Could you check a few things on this model? Use its own coordinates, in mm. A direction names the side the tool comes from. Coordinates: 2 decimals unless noted, no trailing zeros. Loops run counter-clockwise (first coordinate to the right, second up) from the corner with the lowest first, then second, coordinate; pieces in that order, holes last. Notation, with made-up numbers: (78, 14) -> (91, 14) arc R15 ccw to (91, 33) -> close; hole circle Ø3 at (18.25, -39). An arc over 180 degrees is marked (long way). One line per question, with ' | ' between items.
from build123d import *

# Parameters (mm, degrees)
PAD_DEPTH                                 = 3
EXTRUDE_DEPTH                             = 3
EXTRUDE_ONTO_INVOLUTEGEAR_PLACEMENT_ANGLE = -15
SKETCH001_R                               = 3.25
POCKET_DEPTH                              = 1.5
SKETCH002_R                               = 1
POCKET001_DEPTH                           = 3.001
SKETCH003_R                               = 0.75
POCKET002_DEPTH                           = 3.001


with BuildPart() as claw_body:
    # Sketch → Pad (new body)
    with BuildSketch(Plane.XY):
        with BuildLine():
            ThreePointArc((2.197615, -4.7128), (3.983431, 3.342496), (-4.259591, 2.982597))
            Line((-5.488319, 3.842962), (-4.259591, 2.982597))
            Line((-5.488319, 3.842962), (-21.76598, 2.989886))
            ThreePointArc((-22.627333, 3.40073), (-22.248827, 3.08593), (-21.76598, 2.989886))
            Line((-22.627333, 3.40073), (-37.615857, 24.030664))
            ThreePointArc((-37.625992, 25.192025), (-37.806802, 24.609722), (-37.615857, 24.030664))
            Line((-37.625992, 25.192025), (-21.393779, 48.374028))
            ThreePointArc((-21.393779, 48.374028), (-21.125112, 49.710122), (-21.924071, 50.814201))
            ThreePointArc((-21.924071, 50.814201), (-25.071791, 51.496726), (-28.008332, 50.173585))
            Line((-28.008332, 50.173585), (-51.085112, 29.027611))
            ThreePointArc((-51.085112, 29.027611), (-52.688135, 25.777003), (-51.673928, 22.297417))
            Line((-51.673928, 22.297417), (-26.288576, -10.785417))
            ThreePointArc((-26.288576, -10.785417), (-24.440562, -12.203448), (-22.131119, -12.507492))
            Line((-22.131119, -12.507492), (-0.517621, -9.662021))
            ThreePointArc((-0.517621, -9.662021), (2.094081, -7.875425), (2.197615, -4.7128))
        make_face()
    extrude(amount=PAD_DEPTH)


with BuildPart() as horn_drill:
    # InvoluteGear as drawn → Extrude (new)
    with BuildSketch(Plane.XY):
        with BuildLine():
            Line((4.810602, -1.107072), (6.405135, -1.472675))
            add(Edge.make_bspline(
                [(6.405135, -1.472675), (6.508382, -1.483345), (6.922829, -1.512197), (7.670072, -1.341281), (8.519169, -0.723794)],
                knots=[0, 0, 0, 0, 0, 1, 1, 1, 1, 1], degree=4))
            ThreePointArc((8.519169, -0.723794), (8.54986, 0), (8.519169, 0.723794))
            add(Edge.make_bspline(
                [(8.519169, 0.723794), (7.670072, 1.341281), (6.922829, 1.512197), (6.508382, 1.483345), (6.405135, 1.472675)],
                knots=[0, 0, 0, 0, 0, 1, 1, 1, 1, 1], degree=4))
            Line((6.405135, 1.472675), (4.810602, 1.107072))
            ThreePointArc((4.810602, 1.107072), (4.31977, 1.170473), (3.988644, 1.538293))
            ThreePointArc((3.988644, 1.538293), (3.851642, 1.854853), (3.689565, 2.159338))
            ThreePointArc((3.689565, 2.159338), (3.608445, 2.647554), (3.864905, 3.070832))
            Line((3.864905, 3.070832), (5.14492, 4.089539))
            add(Edge.make_bspline(
                [(5.14492, 4.089539), (5.217636, 4.163608), (5.498597, 4.469646), (5.830867, 5.160429), (5.8775, 6.209276)],
                knots=[0, 0, 0, 0, 0, 1, 1, 1, 1, 1], degree=4))
            ThreePointArc((5.8775, 6.209276), (5.330751, 6.68455), (4.74573, 7.111832))
            add(Edge.make_bspline(
                [(4.74573, 7.111832), (3.733556, 6.832978), (3.13403, 6.355326), (2.898184, 6.013309), (2.842153, 5.925934)],
                knots=[0, 0, 0, 0, 0, 1, 1, 1, 1, 1], degree=4))
            Line((2.842153, 5.925934), (2.133817, 4.451328))
            ThreePointArc((2.133817, 4.451328), (1.77822, 4.10711), (1.284193, 4.077557))
            ThreePointArc((1.284193, 4.077557), (0.951277, 4.167817), (0.612168, 4.230943))
            ThreePointArc((0.612168, 4.230943), (0.179887, 4.471919), (0.008856, 4.936337))
            Line((0.008856, 4.936337), (0.010475, 6.572246))
            add(Edge.make_bspline(
                [(0.010475, 6.572246), (-0.002097, 6.675279), (-0.066191, 7.085755), (-0.3991, 7.77623), (-1.190047, 8.466635)],
                knots=[0, 0, 0, 0, 0, 1, 1, 1, 1, 1], degree=4))
            ThreePointArc((-1.190047, 8.466635), (-1.902523, 8.335497), (-2.60134, 8.144516))
            add(Edge.make_bspline(
                [(-2.60134, 8.144516), (-3.014403, 7.179304), (-3.014758, 6.412764), (-2.894406, 6.015128), (-2.861029, 5.916844)],
                knots=[0, 0, 0, 0, 0, 1, 1, 1, 1, 1], degree=4))
            Line((-2.861029, 5.916844), (-2.149775, 4.443643))
            ThreePointArc((-2.149775, 4.443643), (-2.102366, 3.951009), (-2.387281, 3.546338))
            ThreePointArc((-2.387281, 3.546338), (-2.665419, 3.34233), (-2.926204, 3.116562))
            ThreePointArc((-2.926204, 3.116562), (-3.384129, 2.928837), (-3.853862, 3.08468))
            Line((-3.853862, 3.08468), (-5.131858, 4.105918))
            add(Edge.make_bspline(
                [(-5.131858, 4.105918), (-5.220251, 4.160329), (-5.581136, 4.366146), (-6.328536, 4.536371), (-7.361464, 4.348444)],
                knots=[0, 0, 0, 0, 0, 1, 1, 1, 1, 1], degree=4))
            ThreePointArc((-7.361464, 4.348444), (-7.703158, 3.709645), (-7.989548, 3.044213))
            add(Edge.make_bspline(
                [(-7.989548, 3.044213), (-7.492456, 2.119467), (-6.893372, 1.64126), (-6.507449, 1.487434), (-6.409797, 1.45225)],
                knots=[0, 0, 0, 0, 0, 1, 1, 1, 1, 1], degree=4))
            Line((-6.409797, 1.45225), (-4.814543, 1.089804))
            ThreePointArc((-4.814543, 1.089804), (-4.399827, 0.819718), (-4.261084, 0.344654))
            ThreePointArc((-4.261084, 0.344654), (-4.275, 0), (-4.261084, -0.344654))
            ThreePointArc((-4.261084, -0.344654), (-4.399827, -0.819718), (-4.814543, -1.089804))
            Line((-4.814543, -1.089804), (-6.409797, -1.45225))
            add(Edge.make_bspline(
                [(-6.409797, -1.45225), (-6.507449, -1.487434), (-6.893372, -1.64126), (-7.492456, -2.119467), (-7.989548, -3.044213)],
                knots=[0, 0, 0, 0, 0, 1, 1, 1, 1, 1], degree=4))
            ThreePointArc((-7.989548, -3.044213), (-7.703158, -3.709645), (-7.361464, -4.348444))
            add(Edge.make_bspline(
                [(-7.361464, -4.348444), (-6.328536, -4.536371), (-5.581136, -4.366146), (-5.220251, -4.160329), (-5.131858, -4.105918)],
                knots=[0, 0, 0, 0, 0, 1, 1, 1, 1, 1], degree=4))
            Line((-5.131858, -4.105918), (-3.853862, -3.08468))
            ThreePointArc((-3.853862, -3.08468), (-3.384129, -2.928837), (-2.926204, -3.116562))
            ThreePointArc((-2.926204, -3.116562), (-2.665419, -3.34233), (-2.387281, -3.546338))
            ThreePointArc((-2.387281, -3.546338), (-2.102366, -3.951009), (-2.149775, -4.443643))
            Line((-2.149775, -4.443643), (-2.861029, -5.916844))
            add(Edge.make_bspline(
                [(-2.861029, -5.916844), (-2.894406, -6.015128), (-3.014758, -6.412764), (-3.014403, -7.179304), (-2.60134, -8.144516)],
                knots=[0, 0, 0, 0, 0, 1, 1, 1, 1, 1], degree=4))
            ThreePointArc((-2.60134, -8.144516), (-1.902523, -8.335497), (-1.190047, -8.466635))
            add(Edge.make_bspline(
                [(-1.190047, -8.466635), (-0.3991, -7.77623), (-0.066191, -7.085755), (-0.002097, -6.675279), (0.010475, -6.572246)],
                knots=[0, 0, 0, 0, 0, 1, 1, 1, 1, 1], degree=4))
            Line((0.010475, -6.572246), (0.008856, -4.936337))
            ThreePointArc((0.008856, -4.936337), (0.179887, -4.471919), (0.612168, -4.230943))
            ThreePointArc((0.612168, -4.230943), (0.951277, -4.167817), (1.284193, -4.077557))
            ThreePointArc((1.284193, -4.077557), (1.77822, -4.10711), (2.133817, -4.451328))
            Line((2.133817, -4.451328), (2.842153, -5.925934))
            add(Edge.make_bspline(
                [(2.842153, -5.925934), (2.898184, -6.013309), (3.13403, -6.355326), (3.733556, -6.832978), (4.74573, -7.111832)],
                knots=[0, 0, 0, 0, 0, 1, 1, 1, 1, 1], degree=4))
            ThreePointArc((4.74573, -7.111832), (5.330751, -6.68455), (5.8775, -6.209276))
            add(Edge.make_bspline(
                [(5.8775, -6.209276), (5.830867, -5.160429), (5.498597, -4.469646), (5.217636, -4.163608), (5.14492, -4.089539)],
                knots=[0, 0, 0, 0, 0, 1, 1, 1, 1, 1], degree=4))
            Line((5.14492, -4.089539), (3.864905, -3.070832))
            ThreePointArc((3.864905, -3.070832), (3.608445, -2.647554), (3.689565, -2.159338))
            ThreePointArc((3.689565, -2.159338), (3.851642, -1.854853), (3.988644, -1.538293))
            ThreePointArc((3.988644, -1.538293), (4.31977, -1.170473), (4.810602, -1.107072))
        make_face()
    extrude(amount=EXTRUDE_DEPTH)


with BuildPart() as horn_drill_1:
    # Extrude onto InvoluteGear placement: moved
    add(horn_drill.part.rotate(Axis((0, 0, 0), (0, 0, 1)), EXTRUDE_ONTO_INVOLUTEGEAR_PLACEMENT_ANGLE))

    # Fusion: union claw-body
    add(claw_body.part)

    # Sketch001 → Pocket (cut)
    with BuildSketch(Plane.XY.offset(3)):
        Circle(SKETCH001_R)
    extrude(amount=-POCKET_DEPTH, mode=Mode.SUBTRACT)

    # Sketch002 → Pocket001 (cut, through all)
    with BuildSketch(Plane(origin=(0, 0, 0), x_dir=(1, 0, 0), z_dir=(0, 0, -1))):
        Circle(SKETCH002_R)
    extrude(amount=-POCKET001_DEPTH, mode=Mode.SUBTRACT)

    # Sketch003 → Pocket002 (cut, through all)
    with BuildSketch(Plane.XY.offset(3)):
        with Locations((-6.714559, -2.989514)):
            Circle(SKETCH003_R)
    extrude(amount=-POCKET002_DEPTH, mode=Mode.SUBTRACT)


solid = horn_drill_1.part
1) We'd pull the mould along X, two halves only. Please class faces 1 (the face through (-30.017, 13.571, 1.479)), 2 (the face through (-11.476, -11.105, 1.479)), 3 (the face through (-39.385, 39.749, 1.479)): pulls with the +X half, pulls with the -X half, needs draft (parallel to the pull), parting line crosses it, or undercut.
Data:
face 1: undercut | face 2: pulls with the +X half | face 3: pulls with the -X half
2) I'm going to push flat-ended pins straight in: pin 1 Ø1 at (x, z) = (-19, 1.5) entering from +Y; pin 2 Ø1.5 at (y, z) = (11.5, 1.5) entering from -X; pin 3 Ø3 at (x, y) = (-32, 28.5) entering from -Z; pin 4 Ø1.5 at (y, z) = (0, 2.5) entering from -X. Where does each tip first touch, or does it pass through?
Data:
pin 1: y = 3.16 | pin 2: x = -43.96 | pin 3: through | pin 4: x = -35.14
3) If we section it at C-C on y = 44.5: Please give me the cut outline in (x, z), and give its area (3 significant figures).
Data:
outline: (-34.2, 0) -> (-24.11, 0) -> (-24.11, 3) -> (-34.2, 3) -> close | area: 30.3 mm²
4) I need wall thicknesses on line 1 along Y through (x, z) = (0, 1.2); line 2 along Y through (x, z) = (-37, 0.3); line 3 along X through (y, z) = (35, 2.65). Which ranges of each line are inside material? Lowest first, please. Write a range as from..to.
Data:
line 1: -9.55..-1, 1..8.55 | line 2: 3.17..23.18, 26.09..41.93 | line 3: -44.57..-30.76
5) On a 3-axis mill with a long thin cutter (end or side, diameter ignored), from which of +Z, -Z, +X, -X, +Y, -Y can I reach the whole of each face in a straight line? I mean faces 4 (the face through (-39.16, 5.99, 1.48)), 5 (the face through (1, 1, 1.5)), 6 (the face through (3.931, -3.404, 1.479)), 7 (the face through (5.89, -0.21, 1.48)), 8 (the face through (-31, 13, 3)). Say none if no direction works.
Data:
face 4: +Z, -Z, -X, -Y | face 5: +Z | face 6: +Z, -Z | face 7: +Z, -Z, +X | face 8: +Z, +X, -X, +Y, -Y
6) If we section it at B-B on x = -19: Please give me the cut outline in (y, z), and give its area (3 significant figures).
Data:
outline: (-12.1, 0) -> (3.13, 0) -> (3.13, 3) -> (-12.1, 3) -> close | area: 45.7 mm²
7) If we section it at A-A on z = 0.9: Give the number of separate pieces and of enclosed holes in the cut face, and give its area (3 significant figures).
Data:
separate pieces: 1 | enclosed holes: 2 | area: 1,200 mm²
